```python
from build123d import *

# Parameters (mm, degrees)
CHAMFER1_SIZE      = 0.75
SKETCH2_OUTSIDE_W  = 21.488
SKETCH2_OUTSIDE_H  = 21.488
CUT_EXTRUDE1_DEPTH = 10


with BuildPart() as part:
    # Sketch1 → Revolve1 (revolve)
    with BuildSketch(Plane.XY):
        Polygon((0, 0), (-3, 0), (-3, 15), (-7, 15), (-7, 19), (0, 19), align=None)
    revolve(axis=Axis((0, 26.2734375, 0), (0, -1, 0)))

    # Chamfer1
    chamfer1_edges = [part.edges().sort_by_distance(p)[0] for p in [
        (7, 19, 0),
        (7, 15, 0),
    ]]
    chamfer(chamfer1_edges, length=CHAMFER1_SIZE)

    # Sketch2 outside → Cut-Extrude1 (cut)
    with BuildSketch(Plane(origin=(0, 19, 0), x_dir=(1, 0, 0), z_dir=(0, 1, 0))):
        Rectangle(SKETCH2_OUTSIDE_W, SKETCH2_OUTSIDE_H)
        Polygon((0.138817894, 6.998623407), (-5.991576715, 3.619531526), (-6.130394609, -3.379091881), (-0.138817894, -6.998623407), (5.991576715, -3.619531526), (6.130394609, 3.379091881), align=None, mode=Mode.SUBTRACT)
    extrude(amount=-CUT_EXTRUDE1_DEPTH, mode=Mode.SUBTRACT)


solid = part.part
```
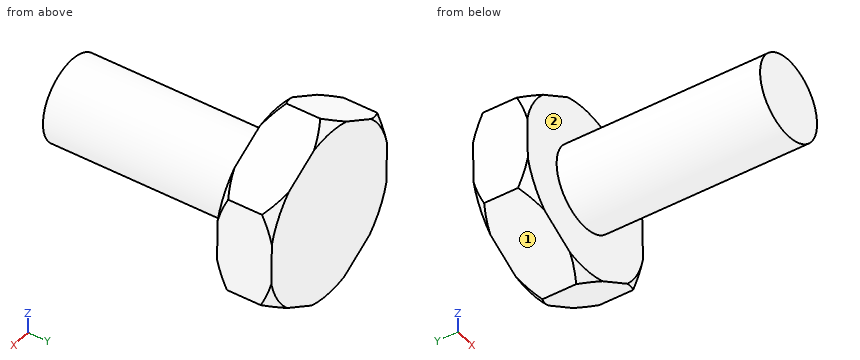
Design review of the part built by this model. Coordinates are the model's own, in mm. Face numbers are marked on the shaded views. A direction names the side the tool comes from. Round coordinates to 2 decimals unless told otherwise and drop trailing zeros. Order: outer loops, then holes, each group sorted by start corner. A loop starts at its lowest first (then second) coordinate and runs counter-clockwise, first axis right, second up. Notation, with made-up numbers: (34.25, -24.75) - (38.25, -24.75) arc R20 ccw to (38.25, -7.75) - close; hole circle Ø9 at (83.5, 58). An arc over 180 degrees is marked (long way). Return JSON: item names as keys, results as strings.
Q1. Consider section A-A on x = 2.5. Write out the cut boundary in (y, z), plus the area to 3 significant figures.
Computed values:
{"outline": "(0, -1.66) - (15, -1.66) - (15, -5.57) - (19, -5.57) - (19, 5.54) - (15, 5.54) - (15, 1.66) - (0, 1.66) - close", "area": "94.2 mm2"}
Q2. Consider section B-B on y = 7.5. Write out the cut boundary in (x, z), plus the area to 3 significant figures.
Computed values:
{"outline": "circle Ø6 at (0, 0)", "area": "28.3 mm2"}
Q3. Consider section D-D on x = 4. Write out the cut boundary in (y, z).
Computed values:
{"outline": "(15, -4.67) - (19, -4.67) - (19, 4.72) - (15, 4.72) - close"}
Q4. For pin 1 Ø2 at (x, z) = (-4, -5.5) entering from -Y; pin 2 Ø4 at (x, y) = (-4, 16) entering from +Z; pin 3 Ø2 at (x, y) = (-2.5, 8) entering from -Z; pin 4 Ø4 at (x, z) = (-2, 3) entering from -Y, all flat-tipped, find the tip position at first contact; note any pin that passes through.
Computed values:
{"pin 1": "stops at y = 15", "pin 2": "stops at z = 5.87", "pin 3": "stops at z = -2.6", "pin 4": "stops at y = 0"}
Q5. Machinability: for the marked faces 1 and 2, which of the approach directions +Z, -Z, +X, -X, +Y, -Y give a long, thin tool a straight path to every point of the face, cutting with its end or side? Answer none if there is none.
Computed values:
{"face 1": "-Z, -X, +Y, -Y", "face 2": "-Y"}
Q6. Consider section C-C on z = 0. Write out the cut boundary in (x, y).
Computed values:
{"outline": "(-6.06, 15) - (-3, 15) - (-3, 0) - (3, 0) - (3, 15) - (6.06, 15) - (6.06, 19) - (-6.06, 19) - close"}
Q7. Wall thickness on L1, parallel to Y at x = 4.25, z = -0.5; L2, parallel to X at y = 9, z = 0.75; L3, parallel to Z at x = 2.25, y = 13.5: over which ranges is each line inside the solid? List them lowest first. Write a range as [from, to].
Computed values:
{"L1": "y = [15, 19]", "L2": "x = [-2.9, 2.9]", "L3": "z = [-1.98, 1.98]"}
